Design review of the part shown in the three views and the two pictorial views. Dimensions are in mm from the part's minimum x, y and z. A direction names the side the tool comes from. Coordinates: 2 decimals unless noted, no trailing zeros. Loops run counter-clockwise (first coordinate to the right, second up) from the corner with the lowest first, then second, coordinate; pieces in that order, holes last. Notation, with made-up numbers: (3.25, 11.5) - (34.25, 11.5) arc R19 cw to (34.25, 23.5) - close; hole circle Ø11 at (-35.75, 15.25). An arc over 180 degrees is marked (long way). One line per item, written item: value. Start each with the question number.
1. The part is to be moulded in two halves that separate along Z. For the marked faces 1 and 2, say which applies: released by +Z, released by -Z, zero draft, split by the parting line, or undercut.
2. To check wall thickness, follow line 1 (Y direction, x = 12.25, z = 2); line 2 (Z direction, x = 10.75, y = 6.25); line 3 (Z direction, x = 1.75, y = 4.5). State the ranges of each line that lie inside material, in increasing order. Write a range as from..to.
3. Take a section at B-B, the plane z = 9. State the section outline as (x, y) points.
4. Take a section at A-A, the plane x = 9.75. State the section outline as (y, z) points.
5. Take a section at C-C, the plane y = 1.5. State the section outline as (x, z) points.
6. Insertion check: pin 1 (1 mm diameter, centred on y = 7.5, z = 20.5, fed in from -X); pin 2 (2 mm diameter, centred on x = 5, y = 7, fed in from +Z); pin 3 (2.5 mm diameter, centred on x = 10, z = 4.5, fed in from +Y); pin 4 (4 mm diameter, centred on x = 15.5, y = 3.5, fed in from -Z). Each pin has a flat end and moves straight along its axis. Give the tip position at first contact, or say it passes through.
7. For the marked faces 3, 4 and 5, list the 3-axis set-ups (+Z, -Z, +X, -X, +Y, -Y) from which the entire face can be reached by the end or side of a thin tool; tool diameter is ignored.
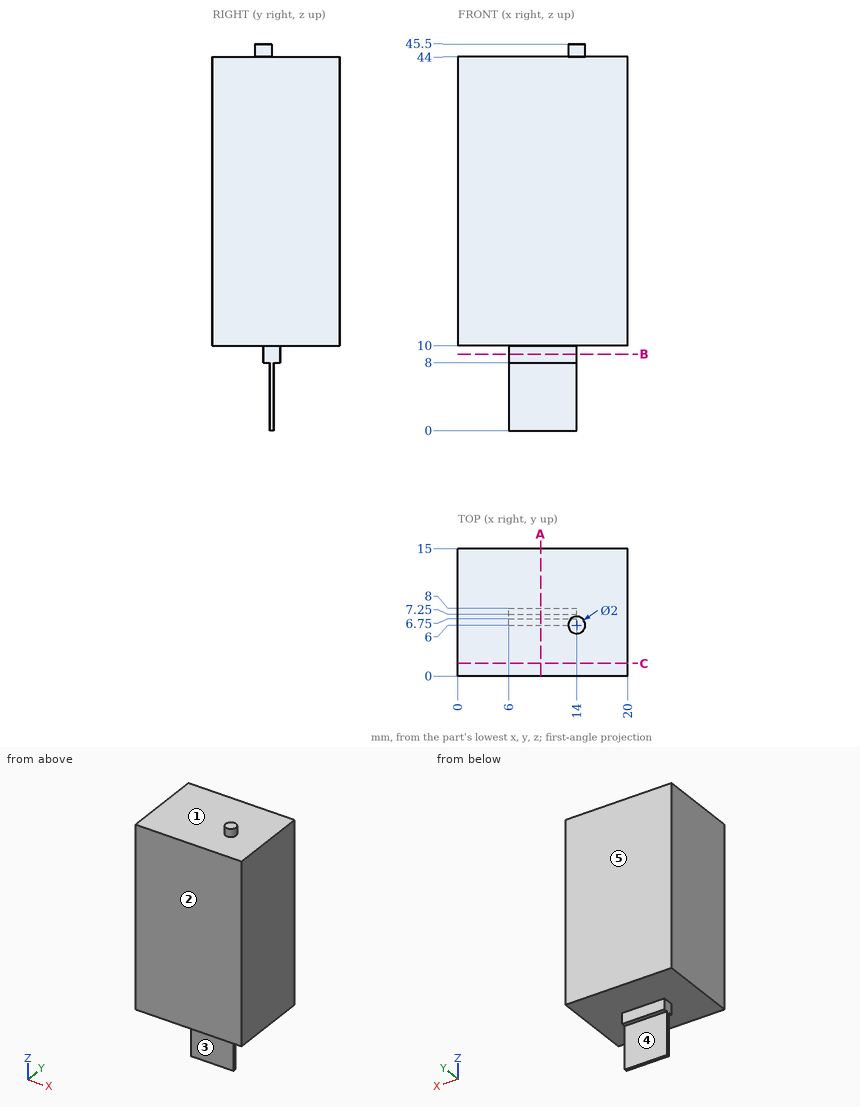
Solutions:
1. face 1: released by +Z
1. face 2: zero draft
2. line 1: 6.75..7.25
2. line 2: 8..44
2. line 3: 10..44
3. outline: (6, 6) - (14, 6) - (14, 8) - (6, 8) - close
4. outline: (0, 10) - (6, 10) - (6, 8) - (6.75, 8) - (6.75, 0) - (7.25, 0) - (7.25, 8) - (8, 8) - (8, 10) - (15, 10) - (15, 44) - (0, 44) - close
5. outline: (0, 10) - (20, 10) - (20, 44) - (0, 44) - close
6. pin 1: x = 0
6. pin 2: z = 44
6. pin 3: y = 7.25
6. pin 4: z = 10
7. face 3: -Z, +X, -X, -Y
7. face 4: -Z, +X, -X, +Y
7. face 5: +Z, -Z, +X, -X, +Y
